Input: dimensioned drawing with shaded views. Units: mm. Origin: part minimum x, y, z. Coordinates: 2 decimals unless noted, no trailing zeros. Loops run counter-clockwise (first coordinate to the right, second up) from the corner with the lowest first, then second, coordinate; pieces in that order, holes last.
Item 1: Line query: probe 1 along Z at (x, y) = (38.1, 1.5) (3 decimals); probe 2 along Z at (x, y) = (44, 1.25); probe 3 along X at (y, z) = (6, 13.5). Output: solid intervals per line, ascending.
Item 2: Section query D-D, the plane y = 3. Return the cut outline in (x, z) (3 decimals).
Item 3: Pin query (flat end, axial travel): pin 1 Ø18.5 at (x, z) = (38.1, 10.16) entering from +Y. Return the tip coordinate at first contact, or that it passes through.
Item 4: Section query B-B, the plane z = 10.16. Return the cut outline in (x, y) (3 decimals), then the cut area to 3 significant figures.
Item 5: Section query A-A, the plane x = 26. Return the cut outline in (y, z).
Item 6: Section query C-C, the plane x = 38.1. Return the cut outline in (y, z) (3 decimals).
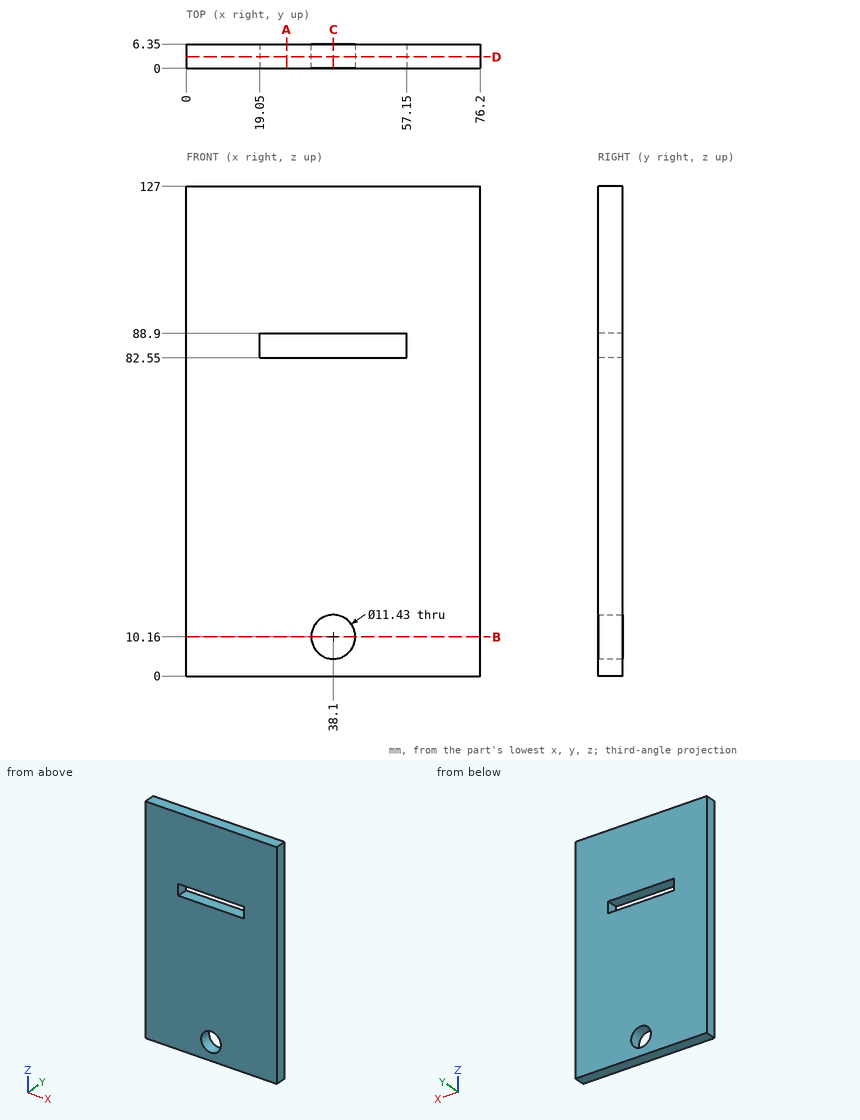
Verdict:
1. probe 1: z = 0 to 4.445, 15.875 to 82.55, 88.9 to 127
1. probe 2: z = 0 to 82.55, 88.9 to 127
1. probe 3: x = 0 to 33.46, 42.74 to 76.2
2. outline: (0, 0) - (76.2, 0) - (76.2, 127) - (0, 127) - close; hole (19.05, 82.55) - (57.15, 82.55) - (57.15, 88.9) - (19.05, 88.9) - close; hole circle Ø11.43 at (38.1, 10.16)
3. pin 1: stops at y = 6.35
4. outline: (0, 0) - (32.385, 0) - (32.385, 6.35) - (0, 6.35) - close; (43.815, 0) - (76.2, 0) - (76.2, 6.35) - (43.815, 6.35) - close
4. area: 411 mm2
5. outline: (0, 0) - (6.35, 0) - (6.35, 82.55) - (0, 82.55) - close; (0, 88.9) - (6.35, 88.9) - (6.35, 127) - (0, 127) - close
6. outline: (0, 0) - (6.35, 0) - (6.35, 4.445) - (0, 4.445) - close; (0, 15.875) - (6.35, 15.875) - (6.35, 82.55) - (0, 82.55) - close; (0, 88.9) - (6.35, 88.9) - (6.35, 127) - (0, 127) - close
